Design review of the part built by this model. Coordinates are the model's own, in mm. A direction names the side the tool comes from. Coordinates: 2 decimals unless noted, no trailing zeros. Loops run counter-clockwise (first coordinate to the right, second up) from the corner with the lowest first, then second, coordinate; pieces in that order, holes last. Notation, with made-up numbers: M -40,-7 L -26,-7 A21 ccw -26,1 Z; hole C 64.25,48 d5. An arc over 180 degrees is marked long. Answer as a JSON object with one key per item and string values. Group by question number.
1. Consider section B-B (z = 9.75). State the section outline as (x, y) points, then the cut area to 3 significant figures.
2. Consider section C-C (x = 6). State the section outline as (y, z) points, then the cut area to 3 significant figures.
3. Consider section A-A (y = 268). State the section outline as (x, z) points.
4. Consider section D-D (y = 121). State the section outline as (x, z) points.
5. Draft analysis for pull direction Y (two halves, no side actions). For faces 3 (the cylindrical face through (19.349, 302.957, 21.535)), 4 (the cylindrical face through (34.297, 311.986, 2.535)), 5 (the flat face through (5.07, 94.07, 11.83)), state which applies: +Y half, -Y half, draft (parallel to the pull), parting line (faces both ways), or undercut.
6. Insertion check: pin 1 (8 mm diameter, centred on y = 32, z = 10.5, fed in from +X); pin 2 (5 mm diameter, centred on y = 129, z = 11, fed in from +X). Each pin has a flat end and moves straight along its axis. Give the tip position at first contact, or say it passes through.
7. To check wall thickness, follow probe 1 along Y at (x, z) = (20, 18.5); probe 2 along Y at (x, z) = (20, 22.4); probe 3 along X at (y, z) = (298, 3.75). State the ranges of each line that lie inside material, in increasing order.
8. Machinability: for faces 1 (the flat face through (24, 303, 5)), 2 (the flat face through (20, 0, 12)), which of the approach directions +Z, -Z, +X, -X, +Y, -Y give a long, thin tool a straight path to every point of the face, cutting with its end or side? Answer none if there is none.
Autodesk Inventor part; units mm, degrees
ref_plane "YZ Plane" through (0, 0, 0) normal (1, 0, 0) x (0, 1, 0)
ref_plane "XZ Plane" through (0, 0, 0) normal (0, 1, 0) x (-1, 0, 0)
ref_plane "XY Plane" through (0, 0, 0) normal (0, 0, 1) x (1, 0, 0)
sketch "スケッチ1" plane through (0, 0, 0) normal (0, 0, 1) x (1, 0, 0)
  line L0 (0, 0) -> (40, 0)
  line L1 (40, 0) -> (40, 318)
  line L2 (40, 318) -> (0, 318)
  line L3 (0, 318) -> (0, 0)
  line L4 (10, 0) -> (0, 190.8114)
  line L5 (40, 190.8114) -> (30, 0)
  dimension "d0" = 40
  dimension "d1" = 318
  dimension "d64" = 20
  dimension "d65" = 10
  dimension "d66" = 87
  dimension "d67" = 87
extrude "押し出し1" add sketch "スケッチ1" along normal blind 24 contours L4 L3 L2 L1 L5 L0
sketch "スケッチ6" plane through (0, 0, 24) normal (0, 0, 1) x (1, 0, 0)
  circle A0 centre (20, 268) radius 5
  line L0 (40, 318) -> (0, 318)
  line L1 (40, 190.8114) -> (40, 318)
  circle A1 centre (20, 20) radius 1.2295
  circle A2 centre (20, 10) radius 1.2295
  line L2 (0, 0) -> (30, 0)
  circle A3 centre (20, 298) radius 5
  point P0 (20, 318)
  point P1 (40, 0)
  dimension "d42" = 10
  dimension "d44" = 20
  dimension "d45" = 2.459
  dimension "d46" = 2.459
  dimension "d47" = 10
  dimension "d48" = 10
  dimension "d49" = 20
  dimension "d50" = 20
  dimension "d53" = 10
  dimension "d54" = 20
  dimension "d55" = 30
  dimension "d56" = 20
extrude "押し出し4" cut sketch "スケッチ6" against normal through all
sketch "スケッチ8" plane through (0, 0, 0) normal (-1, 0, 0) x (0, 0, 1)
  line L0 (0, 318) -> (24, 318)
  line L1 (5, 318) -> (19, 318)
  line L2 (19, 318) -> (19, 288)
  line L3 (19, 288) -> (5, 288)
  line L4 (5, 288) -> (5, 318)
  line L5 (0, 318) -> (0, 0)
  dimension "d57" = 5
  dimension "d58" = 14
  dimension "d59" = 30
extrude "押し出し5" cut sketch "スケッチ8" against normal through all
fillet "フィレット1" radius 20 4 edges at (40, 318, 21.5) (40, 318, 2.5) (0, 318, 2.5) (0, 318, 21.5)
equation "\"d67\" = d66"
equation "\"d45\" = d46"
equation "\"d48\" = d47"
equation "\"d50\" = d49"
properties part number "legparts_06(three)"
Findings below:
{
 "1": {"outline": "M 0,190.81 L 10,0 L 30,0 L 40,190.81 L 40,288 L 0,288 Z; hole C 20,268 d10; hole C 20,10 d2.46; hole C 20,20 d2.46", "area": "9,520 mm^2"},
 "2": {"outline": "M 76.32,0 L 312.28,0 L 312.28,5 L 288,5 L 288,19 L 312.28,19 L 312.28,24 L 76.32,24 Z", "area": "5,320 mm^2"},
 "3": {"outline": "M 0,0 L 15,0 L 15,24 L 0,24 Z; M 25,0 L 40,0 L 40,24 L 25,24 Z"},
 "4": {"outline": "M 3.66,0 L 36.34,0 L 36.34,24 L 3.66,24 Z"},
 "5": {"face 3": "undercut", "face 4": "+Y half", "face 5": "-Y half"},
 "6": {"pin 1": "stops at x = 31.89", "pin 2": "stops at x = 36.89"},
 "7": {"probe 1": "y = 0 to 8.77, 11.23 to 18.77, 21.23 to 263, 273 to 288", "probe 2": "y = 0 to 8.77, 11.23 to 18.77, 21.23 to 263, 273 to 293, 303 to 318", "probe 3": "x = 0 to 15, 25 to 40"},
 "8": {"face 1": "+X, -X, +Y", "face 2": "+Z, -Z, +X, -X, -Y"}
}
